from build123d import *

# Parameters (mm, degrees)
BOSS_EXTRUDE2_DEPTH = 2.54


with BuildPart() as part:
    # Sketch3 → Boss-Extrude2 (new body)
    with BuildSketch(Plane(origin=(0, 0, 0), x_dir=(1, 0, 0), z_dir=(0, 1, 0))):
        Polygon((13.676923077, 25.4), (25.4, 0), (22.922075321, 0), (19.167027244, 8.141025641), (7.652564103, 8.141025641), (3.790665064, 0), (1.302564103, 0), (13.351282051, 25.4), align=None)
        Polygon((13.488661859, 20.449238782), (8.888982372, 10.746153846), (17.966225962, 10.746153846), align=None, mode=Mode.SUBTRACT)
    extrude(amount=BOSS_EXTRUDE2_DEPTH)


solid = part.part
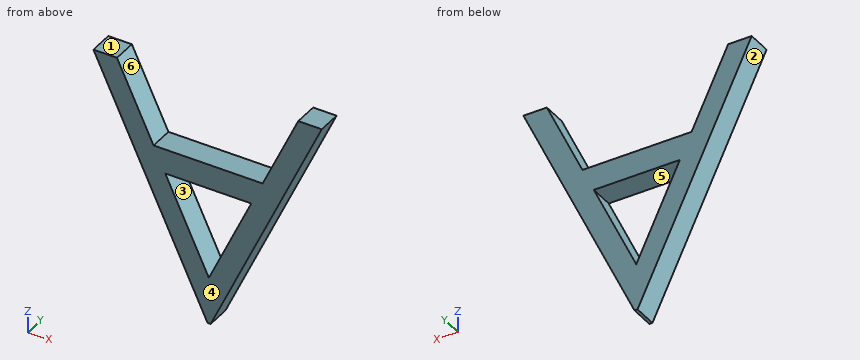
Check sheet for the modelled part. Datum: model origin and axes. Units: mm. Face numbers are marked on the shaded views. A direction names the side the tool comes from. Round coordinates to 2 decimals unless told otherwise and drop trailing zeros. Loops run counter-clockwise (first coordinate to the right, second up) from the corner with the lowest first, then second, coordinate; pieces in that order, holes last.
1. Sectioned sample at A-A on x = 17. Record the boundary of the cut face in (y, z), and give its area (3 significant figures).
2. Gauge pin test, flat ends, axial feed: pin 1 Ø1 at (x, y) = (11.5, 1) entering from -Z; pin 2 Ø1 at (x, y) = (10, 2) entering from -Z; pin 3 Ø0.8 at (x, y) = (16, 1) entering from +Z. Record the tip position at first contact, or that the pin passes through.
3. Scan lines: probe 1 along X at (y, z) = (2.35, -3.75); probe 2 along X at (y, z) = (2.35, -17); probe 3 along X at (y, z) = (1, -9). Record each from-to range of solid material in increasing order.
4. Sectioned sample at B-B on y = 1.85. Record the boundary of the cut face in (x, z).
5. Set-up check for the marked faces 4, 5 and 6: record each of +Z, -Z, +X, -X, +Y, -Y from which the full face is reachable in a straight line by a thin tool's end or side.
6. Sectioned sample at D-D on z = -8.75. Record the boundary of the cut face in (x, y), and give its area (3 significant figures).
7. Sectioned sample at C-C on z = -3.5. Record the boundary of the cut face in (x, y).
8. Mould release check, pull along X, two halves, no side actions. Record for the marked faces 1, 2 and 3: released by +X, released by -X, zero draft, split by the parting line, or undercut.
Recorded:
1. outline: (0, -18.2) - (2.54, -18.2) - (2.54, -12.84) - (0, -12.84) - close; (0, -10.75) - (2.54, -10.75) - (2.54, -8.14) - (0, -8.14) - close
1. area: 20.2 mm2
2. pin 1: stops at z = -22.55
2. pin 2: stops at z = -19.39
2. pin 3: stops at z = -8.14
3. probe 1: x = 3.08 to 5.57, 21.19 to 23.67
3. probe 2: x = 9.37 to 11.85, 15.08 to 17.55
3. probe 3: x = 5.57 to 21.25
4. outline: (1.3, 0) - (13.35, -25.4) - (13.68, -25.4) - (25.4, 0) - (22.92, 0) - (19.17, -8.14) - (7.65, -8.14) - (3.79, 0) - close; hole (8.89, -10.75) - (13.49, -20.45) - (17.97, -10.75) - close
5. face 4: +Z, -Z, +X, -X, -Y
5. face 5: +Y, -Y
5. face 6: +Z, +Y, -Y
6. outline: (5.45, 0) - (21.36, 0) - (21.36, 2.54) - (5.45, 2.54) - close
6. area: 40.4 mm2
7. outline: (2.96, 0) - (5.45, 0) - (5.45, 2.54) - (2.96, 2.54) - close; (21.31, 0) - (23.78, 0) - (23.78, 2.54) - (21.31, 2.54) - close
8. face 1: zero draft
8. face 2: released by -X
8. face 3: undercut
